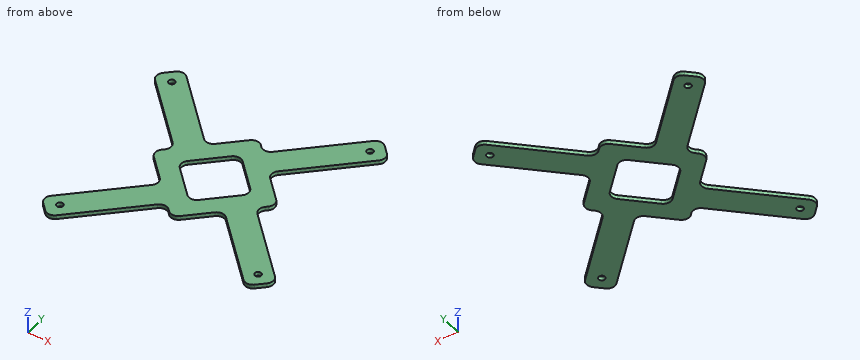
from build123d import *

# Parameters (mm, degrees)
SKETCH2_R           = 1.6
BOSS_EXTRUDE1_DEPTH = 2


with BuildPart() as part:
    # Sketch2 → Boss-Extrude1 (new body)
    with BuildSketch(Plane(origin=(0, 0, 70.507785861), x_dir=(-1, 0, 0), z_dir=(0, 0, -1))):
        with BuildLine():
            Line((-109.491735006, -65.754238005), (-99.238686679, -55.501189677))
            ThreePointArc((-99.238686679, -55.501189677), (-98.067113804, -52.672762553), (-99.238686679, -49.844335428))
            Line((-99.238686679, -49.844335428), (-129.24116868, -19.841853427))
            ThreePointArc((-129.24116868, -19.841853427), (-130.412741556, -17.013426302), (-129.24116868, -14.184999177))
            Line((-129.24116868, -14.184999177), (-125.564213418, -10.508043915))
            ThreePointArc((-125.564213418, -10.508043915), (-122.735786293, -9.33647104), (-119.907359169, -10.508043915))
            Line((-119.907359169, -10.508043915), (-89.904877167, -40.510525916))
            ThreePointArc((-89.904877167, -40.510525916), (-87.076450042, -41.682098792), (-84.248022918, -40.510525916))
            Line((-84.248022918, -40.510525916), (-83.328784102, -39.591287101))
            ThreePointArc((-83.328784102, -39.591287101), (-80.500356977, -38.419714226), (-77.671929853, -39.591287101))
            Line((-77.671929853, -39.591287101), (-67.418881525, -49.844335428))
            ThreePointArc((-67.418881525, -49.844335428), (-64.590454401, -51.015908303), (-61.762027276, -49.844335428))
            Line((-61.762027276, -49.844335428), (-31.759545275, -19.841853427))
            ThreePointArc((-31.759545275, -19.841853427), (-28.93111815, -18.670280551), (-26.102691025, -19.841853427))
            Line((-26.102691025, -19.841853427), (-22.425735763, -23.518808689))
            ThreePointArc((-22.425735763, -23.518808689), (-21.254162888, -26.347235813), (-22.425735763, -29.175662938))
            Line((-22.425735763, -29.175662938), (-52.428217764, -59.17814494))
            ThreePointArc((-52.428217764, -59.17814494), (-53.59979064, -62.006572064), (-52.428217764, -64.834999189))
            Line((-52.428217764, -64.834999189), (-51.508978949, -65.754238005))
            ThreePointArc((-51.508978949, -65.754238005), (-50.337406074, -68.582665129), (-51.508978949, -71.411092254))
            Line((-51.508978949, -71.411092254), (-61.762027276, -81.664140581))
            ThreePointArc((-61.762027276, -81.664140581), (-62.933600151, -84.492567706), (-61.762027276, -87.320994831))
            Line((-61.762027276, -87.320994831), (-31.759545275, -117.323476832))
            ThreePointArc((-31.759545275, -117.323476832), (-30.587972399, -120.151903957), (-31.759545275, -122.980331082))
            Line((-31.759545275, -122.980331082), (-35.436500537, -126.657286344))
            ThreePointArc((-35.436500537, -126.657286344), (-38.264927661, -127.828859219), (-41.093354786, -126.657286344))
            Line((-41.093354786, -126.657286344), (-71.095836788, -96.654804343))
            ThreePointArc((-71.095836788, -96.654804343), (-73.924263912, -95.483231467), (-76.752691037, -96.654804343))
            Line((-76.752691037, -96.654804343), (-77.671929853, -97.574043158))
            ThreePointArc((-77.671929853, -97.574043158), (-80.500356977, -98.745616033), (-83.328784102, -97.574043158))
            Line((-83.328784102, -97.574043158), (-93.581832429, -87.320994831))
            ThreePointArc((-93.581832429, -87.320994831), (-96.410259554, -86.149421956), (-99.238686679, -87.320994831))
            Line((-99.238686679, -87.320994831), (-129.24116868, -117.323476832))
            ThreePointArc((-129.24116868, -117.323476832), (-132.069595805, -118.495049708), (-134.89802293, -117.323476832))
            Line((-134.89802293, -117.323476832), (-138.574978192, -113.64652157))
            ThreePointArc((-138.574978192, -113.64652157), (-139.746551067, -110.818094445), (-138.574978192, -107.989667321))
            Line((-138.574978192, -107.989667321), (-108.572496191, -77.987185319))
            ThreePointArc((-108.572496191, -77.987185319), (-107.400923315, -75.158758194), (-108.572496191, -72.33033107))
            Line((-108.572496191, -72.33033107), (-109.491735006, -71.411092254))
            ThreePointArc((-109.491735006, -71.411092254), (-110.663307881, -68.582665129), (-109.491735006, -65.754238005))
        make_face()
        with Locations((-132.055025121, -110.832665129)):
            Circle(SKETCH2_R, mode=Mode.SUBTRACT)
        with Locations((-28.945688834, -26.332665129)):
            Circle(SKETCH2_R, mode=Mode.SUBTRACT)
        with Locations((-122.750356977, -17.027996986)):
            Circle(SKETCH2_R, mode=Mode.SUBTRACT)
        with Locations((-38.250356977, -120.137333273)):
            Circle(SKETCH2_R, mode=Mode.SUBTRACT)
        with BuildLine():
            Line((-96.339548876, -65.754238005), (-83.328784102, -52.743473231))
            ThreePointArc((-83.328784102, -52.743473231), (-80.500356977, -51.571900356), (-77.671929853, -52.743473231))
            Line((-77.671929853, -52.743473231), (-64.661165079, -65.754238005))
            ThreePointArc((-64.661165079, -65.754238005), (-63.489592204, -68.582665129), (-64.661165079, -71.411092254))
            Line((-64.661165079, -71.411092254), (-77.671929853, -84.421857028))
            ThreePointArc((-77.671929853, -84.421857028), (-80.500356977, -85.593429903), (-83.328784102, -84.421857028))
            Line((-83.328784102, -84.421857028), (-96.339548876, -71.411092254))
            ThreePointArc((-96.339548876, -71.411092254), (-97.511121751, -68.582665129), (-96.339548876, -65.754238005))
        make_face(mode=Mode.SUBTRACT)
    extrude(amount=BOSS_EXTRUDE1_DEPTH)


solid = part.part
Can you work these out from the model? Positions are in its coordinate system, mm. Give positions to 0.01 mm unless a question says otherwise; leave off trailing zeros. Loops run counter-clockwise (first coordinate to the right, second up) from the corner with the lowest first, then second, coordinate; pieces in that order, holes last. Notation, with made-up numbers: M 11.5,72.25 L 31.5,72.25 A14 ccw 31.5,81.25 Z; hole C 9,-26 d9. An arc over 180 degrees is marked long. One line per item, written item: value. Start each with the question number.
1) If we section it at C-C, the plane z = 69.4: Give the number of separate pieces and of enclosed holes in the cut face, and give its area (3 significant figures).
2) If we section it at A-A, the plane y = -34: Write out the boundary of the cut face in (x, z), and give its area (3 significant figures).
3) If I drill on line 1 (Y direction, x = 108, z = 68.75); line 2 (Y direction, x = 122, z = 69.3); line 3 (Y direction, x = 102, z = 70.3), over which ranges is the centre line in solid material (lowest first)? Write a range as [from, to].
4) If we section it at B-B, the plane x = 44.5: Write out the boundary of the cut face in (y, z).
Completed:
1. separate pieces: 1
1. enclosed holes: 5
1. area: 3,960 mm^2
2. outline: M 27.25,68.51 L 45.92,68.51 L 45.92,70.51 L 27.25,70.51 Z; M 96.42,68.51 L 115.08,68.51 L 115.08,70.51 L 96.42,70.51 Z
2. area: 74.7 mm^2
3. line 1: y = [-96.08, -77.26], [-73.05, -64.26], [-41.08, -22.42]
3. line 2: y = [-110.08, -91.41], [-27.08, -18.44], [-15.61, -9.4]
3. line 3: y = [-90.08, -58.26], [-47.08, -28.42]
4. outline: M -123.25,68.51 L -104.58,68.51 L -104.58,70.51 L -123.25,70.51 Z; M -51.25,68.51 L -32.58,68.51 L -32.58,70.51 L -51.25,70.51 Z
